```python
from build123d import *

# Parameters (mm, degrees)
SKETCH_1_W          = 40
SKETCH_1_H          = 25
EXTRUDE_1_DEPTH     = 20
SKETCH_3_R          = 3
CUT_EXTRUDE_2_DEPTH = 41
SKETCH_2_R          = 4.1
CUT_EXTRUDE_1_DEPTH = 26
SKETCH_4_W          = 25
SKETCH_4_H          = 5
CUT_EXTRUDE_3_DEPTH = 20
SKETCH_5_R          = 4.1
CUT_EXTRUDE_4_DEPTH = 3
SKETCH_6_R          = 1.6
CUT_EXTRUDE_5_DEPTH = 21
SKETCH_7_R          = 1.6
CUT_EXTRUDE_6_DEPTH = 41
SKETCH_8_W          = 25
SKETCH_8_H          = 20
EXTRUDE_2_DEPTH     = 12
SKETCH_9_R          = 1.6
CUT_EXTRUDE_7_DEPTH = 21.0000001
SKETCH_10_R         = 2
CUT_EXTRUDE_8_DEPTH = 26
SKETCH_12_R         = 5
CUT_EXTRUDE_9_DEPTH = 23


with BuildPart() as part:
    # Эскиз1 → Бобышка-Вытянуть1 (new body)
    with BuildSketch(Plane(origin=(0, 0, 0), x_dir=(1, 0, 0), z_dir=(0, 1, 0))):
        Rectangle(SKETCH_1_W, SKETCH_1_H)
    extrude(amount=EXTRUDE_1_DEPTH)

    # Эскиз3 → Вырез-Вытянуть2 (cut, through all)
    with BuildSketch(Plane.ZY.offset(20)):
        with Locations((0, 10)):
            Circle(SKETCH_3_R)
    extrude(amount=-CUT_EXTRUDE_2_DEPTH, mode=Mode.SUBTRACT)

    # Эскиз2 → Вырез-Вытянуть1 (cut)
    with BuildSketch(Plane.ZY.offset(20)):
        with Locations((0, 10)):
            Circle(SKETCH_2_R)
    extrude(amount=-CUT_EXTRUDE_1_DEPTH, mode=Mode.SUBTRACT)

    # Эскиз4 → Вырез-Вытянуть3 (cut)
    with BuildSketch(Plane(origin=(-20, 0, 0), x_dir=(0, 0, -1), z_dir=(1, 0, 0))):
        with Locations((0, 10)):
            Rectangle(SKETCH_4_W, SKETCH_4_H)
    extrude(amount=CUT_EXTRUDE_3_DEPTH, mode=Mode.SUBTRACT)

    # Эскиз5 → Вырез-Вытянуть4 (cut)
    with BuildSketch(Plane(origin=(20, 0, 0), x_dir=(0, 0, -1), z_dir=(1, 0, 0))):
        with Locations((0, 10)):
            Circle(SKETCH_5_R)
    extrude(amount=-CUT_EXTRUDE_4_DEPTH, mode=Mode.SUBTRACT)

    # Эскиз6 → Вырез-Вытянуть5 (cut, through all)
    with BuildSketch(Plane(origin=(0, 20, 0), x_dir=(1, 0, 0), z_dir=(0, 1, 0))):
        with Locations((-15, 0)):
            Circle(SKETCH_6_R)
    extrude(amount=-CUT_EXTRUDE_5_DEPTH, mode=Mode.SUBTRACT)

    # Эскиз7 → Вырез-Вытянуть6 (cut, through all)
    with BuildSketch(Plane.ZY.offset(20)):
        with Locations((-9, 16.5)):
            Circle(SKETCH_7_R)
        with Locations((9, 16.5)):
            Circle(SKETCH_7_R)
        with Locations((-9, 3.5)):
            Circle(SKETCH_7_R)
        with Locations((9, 3.5)):
            Circle(SKETCH_7_R)
    extrude(amount=-CUT_EXTRUDE_6_DEPTH, mode=Mode.SUBTRACT)

    # Эскиз8 → Бобышка-Вытянуть2 (add)
    with BuildSketch(Plane.XY.offset(12.5)):
        with Locations((17.5, 10)):
            Rectangle(SKETCH_8_W, SKETCH_8_H)
    extrude(amount=EXTRUDE_2_DEPTH)

    # Эскиз9 → Вырез-Вытянуть7 (cut, through all)
    with BuildSketch(Plane(origin=(0, 20, 0), x_dir=(1, 0, 0), z_dir=(0, 1, 0))):
        with Locations((14, -21.5)):
            Circle(SKETCH_9_R)
        with Locations((14, 5.5)):
            Circle(SKETCH_9_R)
        with Locations((14, -12.5)):
            Circle(SKETCH_9_R)
    extrude(amount=-CUT_EXTRUDE_7_DEPTH, mode=Mode.SUBTRACT)

    # Эскиз10 → Вырез-Вытянуть8 (cut, through all)
    with BuildSketch(Plane.ZY.offset(-5)):
        with Locations((17.5, 10)):
            Circle(SKETCH_10_R)
    extrude(amount=-CUT_EXTRUDE_8_DEPTH, mode=Mode.SUBTRACT)

    # Эскиз12 → Вырез-Вытянуть9 (cut)
    with BuildSketch(Plane.ZY.offset(20)):
        with Locations((0, 10)):
            Circle(SKETCH_12_R)
    extrude(amount=-CUT_EXTRUDE_9_DEPTH, mode=Mode.SUBTRACT)


solid = part.part
```
Design review of the part built by this model. Coordinates are the model's own, in mm. A direction names the side the tool comes from. Round coordinates to 2 decimals unless told otherwise and drop trailing zeros. Write each loop counter-clockwise with the first axis right and the second up, starting at its lowest first coordinate (ties: lowest second). Pieces come first, ordered by that corner, then holes.
Item 1: We need section D-D on x = 1. Write out the cut boundary in (y, z).
Item 2: For probe 1 along Y at (x, z) = (-10, 5.5); probe 2 along Y at (x, z) = (18.15, 0); probe 3 along Z at (x, y) = (11.5, 4), list the stretches that pass through material, from the lowest coordinate up.
Item 3: For faces 4 (the flat face through (17, 9, 3)), 5 (the cylindrical face through (-9, 7, -4)), 6 (the flat face through (5, 10, 20)), 7 (the flat face through (-10, 12.5, -8)), list the 3-axis set-ups (+Z, -Z, +X, -X, +Y, -Y) from which the entire face can be reached by the end or side of a thin tool; tool diameter is ignored.
Item 4: We need section A-A on y = 3.5. Write out the cut boundary in (x, z).
Item 5: We need section B-B on z = 17.5. Write out the cut boundary in (x, y), and give its area (3 significant figures).
Item 6: The part is to be moulded in two halves that separate along X. For faces 1 (the cylindrical face through (12.4, 10.14, -5.57)), 2 (the flat face through (0, 10, 8)), 3 (the cylindrical face through (17.325, 11.352, 16.026)), say which applies: +X half, -X half, draft (parallel to the pull), parting line (faces both ways), or undercut.
Item 7: Clearance check with flat-ended pins moving along their axes: pin 1 Ø8 at (x, z) = (-1.5, 9) entering from -Y; pin 2 Ø6.5 at (y, z) = (11, 0.5) entering from -X; pin 3 Ø6.5 at (y, z) = (11, 1) entering from +X. State where each tip first meets the part, or that it passes through.
Item 8: We need section C-C on x = -15. Write out the cut boundary in (y, z).
Returned:
1. outline: (0, -12.5) - (20, -12.5) - (20, 12.5) - (0, 12.5) - close; hole circle Ø3.2 at (3.5, -9); hole circle Ø3.2 at (3.5, 9); hole circle Ø10 at (10, 0); hole circle Ø3.2 at (16.5, -9); hole circle Ø3.2 at (16.5, 9)
2. probe 1: y = 0 to 7.5, 12.5 to 20
2. probe 2: y = 0 to 5.9, 14.1 to 20
2. probe 3: z = -12.5 to -10.52, -7.48 to 7.48, 10.52 to 24.5
3. face 4: +X
3. face 5: -X
3. face 6: +Z, -X, +Y, -Y
3. face 7: +Z, -Z, -X
4. outline: (-20, -12.5) - (20, -12.5) - (20, -10.6) - (-20, -10.6) - close; (-20, -7.4) - (20, -7.4) - (20, 7.4) - (-20, 7.4) - close; (-20, 10.6) - (20, 10.6) - (20, 12.5) - (30, 12.5) - (30, 24.5) - (5, 24.5) - (5, 12.5) - (-20, 12.5) - close; hole circle Ø3.2 at (-15, 0); hole circle Ø3.2 at (14, -5.5); hole circle Ø3.2 at (14, 12.5); hole circle Ø3.2 at (14, 21.5)
5. outline: (5, 0) - (30, 0) - (30, 8) - (5, 8) - close; (5, 12) - (30, 12) - (30, 20) - (5, 20) - close
5. area: 400 mm2
6. face 1: undercut
6. face 2: -X half
6. face 3: draft
7. pin 1: stops at y = 0
7. pin 2: stops at x = 3
7. pin 3: stops at x = 20
8. outline: (0, -12.5) - (7.5, -12.5) - (7.5, -4.33) arc R5 cw to (5.26, -1.6) - (0, -1.6) - close; (0, 1.6) - (5.26, 1.6) arc R5 cw to (7.5, 4.33) - (7.5, 12.5) - (0, 12.5) - close; (12.5, -12.5) - (20, -12.5) - (20, -1.6) - (14.74, -1.6) arc R5 cw to (12.5, -4.33) - close; (12.5, 4.33) arc R5 cw to (14.74, 1.6) - (20, 1.6) - (20, 12.5) - (12.5, 12.5) - close; hole circle Ø3.2 at (3.5, -9); hole circle Ø3.2 at (3.5, 9); hole circle Ø3.2 at (16.5, -9); hole circle Ø3.2 at (16.5, 9)
